Study the drawing (mm; zero at the part's minimum x, y, z) and answer. A direction names the side the tool comes from. Coordinates: 2 decimals unless noted, no trailing zeros. Order: outer loops, then holes, each group sorted by start corner. A loop starts at its lowest first (then second) coordinate and runs counter-clockwise, first axis right, second up.
1. Find the intervals of material crossed by probe 1 along X at (y, z) = (11, 64); probe 2 along X at (y, z) = (22.5, 41); probe 3 along Y at (x, z) = (103, 49.5), in increasing order.
2. The part is cut by section C-C, the plane y = 19.5. Give the vertices of the cut face in (x, z), then the cut area to 3 significant figures.
3. The part is cut by section D-D, the plane y = 1.75. Give the vertices of the cut face in (x, z) (1 decimal), then the cut area to 3 significant figures.
4. The part is cut by section B-B, the plane x = 13.5. Give the vertices of the cut face in (y, z).
5. Flat-ended cylindrical pins translate along their axes: pin 1 Ø6 at (y, z) = (6, 26) entering from -X; pin 2 Ø6.5 at (y, z) = (19.5, 68) entering from +X; pin 3 Ø2.5 at (y, z) = (16.5, 69) entering from -X. Find the tip coordinate at first contact, or state that the pin passes through.
6. A tool of negligible diameter and unlimited length cuts with its end or side. For the marked faces 1, 2 and 3, from which of +Z, -Z, +X, -X, +Y, -Y can it reach the whole face along a straight path? Write none if from no direction.
7. The part is cut by section A-A, the plane z = 16.5. Give the vertices of the cut face in (x, y), then the cut area to 3 significant figures.
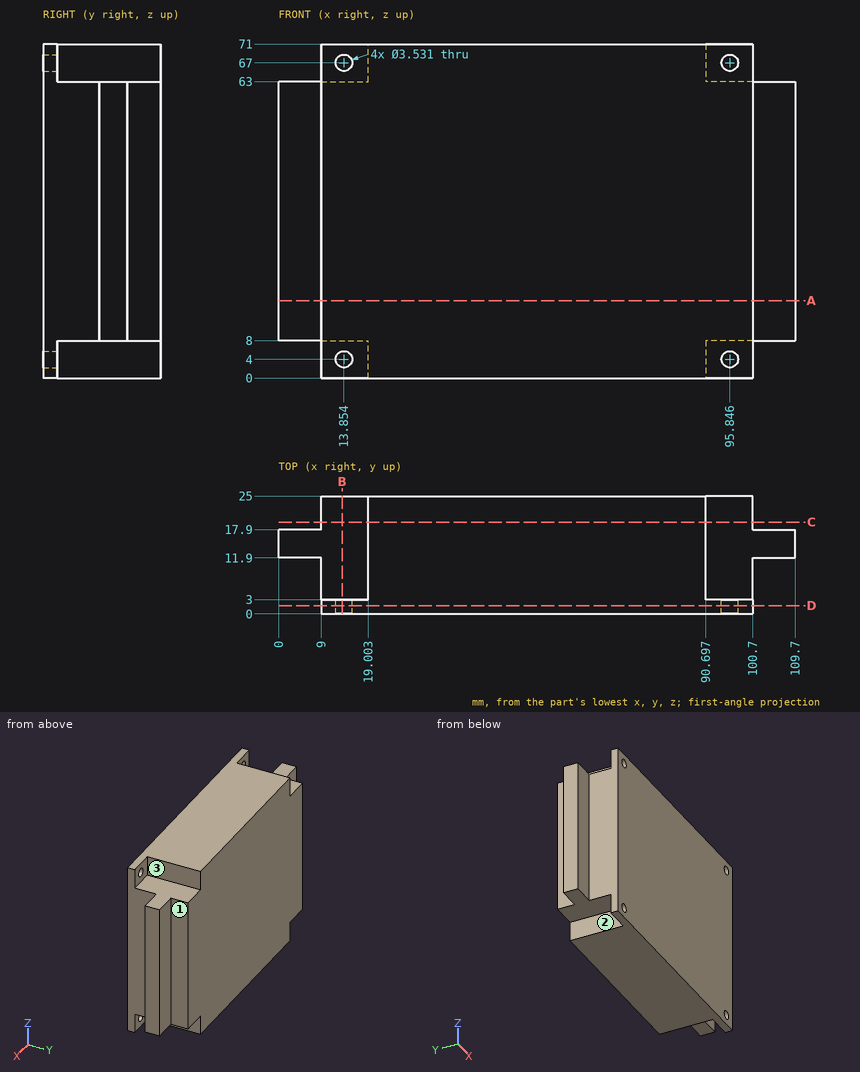
Geometry says:
1. probe 1: x = 19 to 90.7
1. probe 2: x = 9 to 100.7
1. probe 3: y = 11.9 to 17.9
2. outline: (9, 8) - (19, 8) - (19, 0) - (90.7, 0) - (90.7, 8) - (100.7, 8) - (100.7, 63) - (90.7, 63) - (90.7, 71) - (19, 71) - (19, 63) - (9, 63) - close
2. area: 6,190 mm2
3. outline: (9, 0) - (100.7, 0) - (100.7, 71) - (9, 71) - close; hole circle Ø3.5 at (13.9, 4); hole circle Ø3.5 at (13.9, 67); hole circle Ø3.5 at (95.8, 4); hole circle Ø3.5 at (95.8, 67)
3. area: 6,470 mm2
4. outline: (0, 0) - (3, 0) - (3, 2.27) - (0, 2.27) - close; (0, 5.73) - (3, 5.73) - (3, 8) - (25, 8) - (25, 63) - (3, 63) - (3, 65.27) - (0, 65.27) - close; (0, 68.73) - (3, 68.73) - (3, 71) - (0, 71) - close
5. pin 1: stops at x = 9
5. pin 2: stops at x = 90.7
5. pin 3: stops at x = 19
6. face 1: +Z, -Z, +X, +Y
6. face 2: -Z, -X, +Y
6. face 3: +Z, +X, +Y
7. outline: (0, 11.9) - (9, 11.9) - (9, 0) - (100.7, 0) - (100.7, 11.9) - (109.7, 11.9) - (109.7, 17.9) - (100.7, 17.9) - (100.7, 25) - (9, 25) - (9, 17.9) - (0, 17.9) - close
7. area: 2,400 mm2
